Source: CAD feature listing. Evaluate the final solid. Frame: model axes, mm. A direction names the side the tool comes from. Give positions to 0.01 mm unless a question says otherwise; leave off trailing zeros. Loops run counter-clockwise (first coordinate to the right, second up) from the corner with the lowest first, then second, coordinate; pieces in that order, holes last. Notation, with made-up numbers: (10, 67.25) -> (48, 67.25) arc R17 ccw to (48, 77.25) -> close; hole circle Ø10 at (-34, 19). An arc over 180 degrees is marked (long way). Put each result on its own line as item: value.
Autodesk Inventor part; units mm, degrees
ref_plane "YZ Plane" through (0, 0, 0) normal (1, 0, 0) x (0, 1, 0)
ref_plane "XZ Plane" through (0, 0, 0) normal (0, 1, 0) x (-1, 0, 0)
ref_plane "XY Plane" through (0, 0, 0) normal (0, 0, 1) x (1, 0, 0)
sketch "Sketch_1" plane through (0, 0, 0) normal (0, 0, 1) x (1, 0, 0)
  line L0 (137, 0) -> (0, 0)
  line L1 (0, 0) -> (0, 3.5)
  line L2 (0, 3.5) -> (0.5, 4)
  line L3 (0.5, 4) -> (136.5, 4)
  line L4 (136.5, 4) -> (137, 3.5)
  line L5 (137, 3.5) -> (137, 0)
  line L6 (137, 0) -> (0, 0)
revolve "Revolution1" add sketch "Sketch_1" angle 360 about axis through (137, 0, 0) along (1, 0, 0)
sketch "Sketch2" plane through (0, 0, 0) normal (-1, 0, 0) x (0, 0, 1)
  point P0 (0, 0)
hole "Hole1" at (0, 0, 0) direction (1, 0, 0) diameter 3.242 depth 13.0641 tip angle 120 countersink diameter 4 countersink angle 90
sketch "Sketch3" plane through (137, 0, 0) normal (1, 0, 0) x (0, 0, -1)
  point P0 (0, 0)
hole "Hole2" at (137, 0, 0) direction (-1, 0, 0) diameter 3.242 depth 13.0641 tip angle 120 countersink diameter 4 countersink angle 90
properties part number "SFHRW8-137-M4-N4_s" material "鋼、炭素鋼"
(1) Reachability of faces 1 (the cylindrical face through (6.81, 1.438, 0.748)), 2 (the flat face through (137, 2, -2)) from +Z, -Z, +X, -X, +Y, -Y: full face, straight path, thin tool, end or side. Return the list, or none.
Calculated:
face 1: -X
face 2: +Z, -Z, +X, +Y, -Y
(2) Draft query along Y for faces 3 (the flat face through (0, 2, -2)), 4 (the cylindrical face through (130.19, 1.438, -0.748)), 5 (the cylindrical face through (69.452, -0.867, -3.905)). Return one class per face: released by +Y, released by -Y, zero draft, split by the parting line, or undercut.
Calculated:
face 3: zero draft
face 4: undercut
face 5: split by the parting line
(3) Section B-B on x = 97. Return loops of the section in (y, z).
Calculated:
outline: circle Ø8 at (0, 0)
(4) Line query: probe 1 along Z at (x, y) = (4.5, 0); probe 2 along Z at (x, y) = (15, -0.25); probe 3 along Y at (x, z) = (104, -2). Output: solid intervals per line, ascending. Write a range as from..to.
Calculated:
probe 1: z = -4..-1.62, 1.62..4
probe 2: z = -3.99..3.99
probe 3: y = -3.46..3.46
(5) Section A-A on x = 126. Return loops of the section in (y, z), then the cut area to 3 significant figures.
Calculated:
outline: circle Ø8 at (0, 0); hole circle Ø3.24 at (0, 0)
area: 42.0 mm²
(6) First-contact query: P1, Ø1.9, axis at y = 0, z = 0, coming from the -X side; P2, Ø1, axis at x = 49.5, z = 1, coming from the -Y side; P3, Ø3, axis at x = 91, y = -3, coming from the -Z side. Flat tips, straight axial feed; report the tip coordinate or a pass-through.
Calculated:
P1: stops at x = 13.45
P2: stops at y = -3.97
P3: stops at z = -3.71
